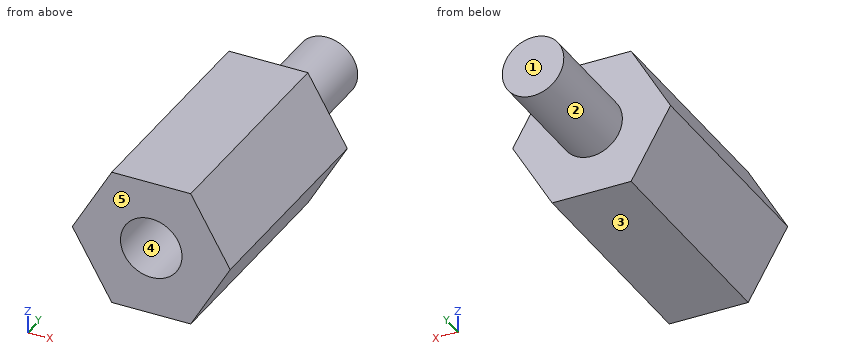
from build123d import *

# Parameters (mm, degrees)
EXTRUDE_1_DEPTH     = 10
SKETCH_2_R          = 1.35
EXTRUDE_2_DEPTH     = 5
SKETCH_3_R          = 1.35
CUT_EXTRUDE_1_DEPTH = 6


with BuildPart() as part:
    # 스케치1 → 보스-돌출1 (new body)
    with BuildSketch(Plane(origin=(0, 0, 0), x_dir=(1, 0, 0), z_dir=(0, 1, 0))):
        Polygon((3.464101615, 0), (1.732050808, 3), (-1.732050808, 3), (-3.464101615, 0), (-1.732050808, -3), (1.732050808, -3), align=None)
    extrude(amount=EXTRUDE_1_DEPTH)

    # 스케치2 → 보스-돌출2 (add)
    with BuildSketch(Plane(origin=(0, 10, 0), x_dir=(1, 0, 0), z_dir=(0, 1, 0))):
        with Locations(Location((0, 0, 0), (0, 0, 270))):
            Circle(SKETCH_2_R)
    extrude(amount=EXTRUDE_2_DEPTH)

    # 스케치3 → 컷-돌출1 (cut)
    with BuildSketch(Plane.XZ):
        with Locations(Location((0, 0, 0), (0, 0, 90))):
            Circle(SKETCH_3_R)
    extrude(amount=-CUT_EXTRUDE_1_DEPTH, mode=Mode.SUBTRACT)


solid = part.part
The model under review builds one solid part; all positions refer to its coordinate system, in mm. Face numbers are marked on the shaded views. A direction names the side the tool comes from. Give positions to 0.01 mm unless a question says otherwise; leave off trailing zeros. Order: outer loops, then holes, each group sorted by start corner. A loop starts at its lowest first (then second) coordinate and runs counter-clockwise, first axis right, second up. Notation, with made-up numbers: M 65.5,25 L 83.5,25 A12 cw 83.5,36 Z; hole C -30,-13 d11. An arc over 180 degrees is marked long. One line per question, with ' | ' between items. Start each with the question number.
1) Consider section C-C, the plane x = 0. Give the boundary of the cut face in (y, z), then the cut area to 3 significant figures.
2) Consider section D-D, the plane y = 6.75. Give the boundary of the cut face in (x, z).
3) Wall thickness on L1, parallel to Y at x = -0.75, z = -2.25; L2, parallel to X at y = 12.75, z = 0; L3, parallel to Y at x = 1, z = 0.75: over which ranges is each line inside the solid? List them lowest first. Write a range as from..to.
4) For the marked faces 1 and 2, list the 3-axis set-ups (+Z, -Z, +X, -X, +Y, -Y) from which the entire face can be reached by the end or side of a thin tool; tool diameter is ignored.
5) Mouldability with a two-part tool opening along Z and no side actions: class the marked faces 3, 4 and 5 as pulls with the +Z half, pulls with the -Z half, needs draft (parallel to the pull), parting line crosses it, or undercut.
6) Clearance check with a flat-ended pin moving along its axis: P1, Ø1, axis at x = -2, z = 2, coming from the +Y side. State where the tip first meets the part, or that it passes through.
7) Consider section A-A, the plane y = 1. Give the boundary of the cut face in (x, z).
8) Consider section B-B, the plane z = -0.5. Give the boundary of the cut face in (x, y), then the cut area to 3 significant figures.
Found:
1) outline: M 0,-3 L 10,-3 L 10,-1.35 L 15,-1.35 L 15,1.35 L 10,1.35 L 10,3 L 0,3 L 0,1.35 L 6,1.35 L 6,-1.35 L 0,-1.35 Z | area: 57.3 mm²
2) outline: M -3.46,0 L -1.73,-3 L 1.73,-3 L 3.46,0 L 1.73,3 L -1.73,3 Z
3) L1: y = 0..10 | L2: x = -1.35..1.35 | L3: y = 6..15
4) face 1: +Z, -Z, +X, -X, +Y | face 2: +Y
5) face 3: pulls with the -Z half | face 4: undercut | face 5: needs draft
6) P1: stops at y = 10
7) outline: M -3.46,0 L -1.73,-3 L 1.73,-3 L 3.46,0 L 1.73,3 L -1.73,3 Z; hole C 0,0 d2.7
8) outline: M -3.18,0 L -1.25,0 L -1.25,6 L 1.25,6 L 1.25,0 L 3.18,0 L 3.18,10 L 1.25,10 L 1.25,15 L -1.25,15 L -1.25,10 L -3.18,10 Z | area: 61.0 mm²
